Autodesk Inventor part; units mm, degrees
ref_plane "YZ Plane" through (0, 0, 0) normal (1, 0, 0) x (0, 1, 0)
ref_plane "XZ Plane" through (0, 0, 0) normal (0, 1, 0) x (-1, 0, 0)
ref_plane "XY Plane" through (0, 0, 0) normal (0, 0, 1) x (1, 0, 0)
sketch "Skizze1" plane through (0, 0, 0) normal (0, 0, 1) x (1, 0, 0)
  line L0 (-210, 0) -> (210, 0)
  line L1 (0, -168) -> (0, 168)
  ellipse E0 centre (0, 0) end of major axis (-150, 0) minor radius 120
  line L2 (0, 120) -> (0, -120) construction
  line L3 (-150, 0) -> (150, 0) construction
  dimension "d0" = 300
  dimension "d1" = 240
extrude "Extrusion1" add sketch "Skizze1" along normal blind 3
sketch "Skizze4" plane through (0, 0, 0) normal (0, 0, -1) x (-1, 0, 0)
  line L0 (210, 0) -> (-210, 0)
  line L1 (0, -168) -> (0, 168)
  line L2 (80, -40) -> (-80, -40)
  line L3 (-80, -40) -> (-80, 40)
  line L4 (-80, 40) -> (80, 40)
  line L5 (80, 40) -> (80, -40)
  line L6 (80, -40) -> (-80, 40) construction
  line L7 (-80, -40) -> (80, 40) construction
  point P0 (0, 0)
  dimension "d25" = 80
  dimension "d26" = 160
hole "Bohrung2" at (80, 40, 0) at (80, -40, 0) at (-80, -40, 0) at (-80, 40, 0) direction (0, 0, 1) diameter 5.2 end through all
sketch "Skizze5" plane through (0, 0, 0) normal (0, 0, -1) x (-1, 0, 0)
  circle A0 centre (0, -70) radius 35
  point P0 (0, 0)
extrude "Extrusion3" cut sketch "Skizze5" against normal through all
sketch "Skizze6" plane through (0, 0, 3) normal (0, 0, 1) x (1, 0, 0)
  line L0 (37.5, -37.5) -> (-37.5, -37.5)
  line L1 (-37.5, -37.5) -> (-37.5, 37.5)
  line L2 (-37.5, 37.5) -> (37.5, 37.5)
  line L3 (37.5, 37.5) -> (37.5, -37.5)
  line L4 (37.5, -37.5) -> (-37.5, 37.5) construction
  line L5 (-37.5, -37.5) -> (37.5, 37.5) construction
  line L6 (50, -50) -> (-50, -50)
  line L7 (-50, -50) -> (-50, 50)
  line L8 (-50, 50) -> (50, 50)
  line L9 (50, 50) -> (50, -50)
  line L10 (50, -50) -> (-50, 50) construction
  line L11 (-50, -50) -> (50, 50) construction
  point P0 (0, 0)
  dimension "d36" = 100
  dimension "d37" = 100
  dimension "d38" = 75
hole "Bohrung3" at (-50, 50, 3) at (-37.5, 37.5, 3) at (37.5, 37.5, 3) at (50, 50, 3) at (50, -50, 3) at (37.5, -37.5, 3) at (-37.5, -37.5, 3) at (-50, -50, 3) direction (0, 0, -1) diameter 5 end through all
equation "\"d37\" = d36"
properties part number "24_0497_0015" material "LCP-Kunststoff"
Source: CAD feature listing. Evaluate the final solid. Frame: model axes, mm. Give positions to 0.01 mm unless a question says otherwise; leave off trailing zeros. Return JSON: item names as keys, results as strings. Group by question number.
1. Mould query, pull axis X, two halves, no side actions, for faces 1 (the face through (-2, 2, 3)), 2 (the face through (4.56, -35.3, 1.48)). Classes: +X half, -X half, draft (parallel to the pull), parting line (faces both ways), or undercut.
2. Pin query (flat end, axial travel): pin 1 Ø1.5 at (x, z) = (-114, 0.5) entering from +Y. Return the tip coordinate at first contact, or that it passes through.
3. Section A-A, the plane z = 1.5. Count the separate pieces of the cut face and the enclosed holes in it, then the cut area to 3 significant figures.
4. Material intervals for line 1 (Y direction, x = -37.5, z = 0.9); line 2 (Y direction, x = 50, z = 2.35); line 3 (X direction, y = 50, z = 1.1), sorted ascending. Write a range as from..to.
Determined:
{
 "1": {"face 1": "draft", "face 2": "undercut"},
 "2": {"pin 1": "stops at y = 78.69"},
 "3": {"separate pieces": "1", "enclosed holes": "13", "area": "52,500 mm2"},
 "4": {"line 1": "y = -116.19..-40, -35..35, 40..116.19", "line 2": "y = -113.14..-52.5, -47.5..47.5, 52.5..113.14", "line 3": "x = -136.36..-52.5, -47.5..47.5, 52.5..136.36"}
}
